Could you check a few things on this drawing? It's one solid part, dimensions in mm from its lowest x, y, z. Give positions to 0.01 mm unless a question says otherwise; leave off trailing zeros. Write each loop counter-clockwise with the first axis right and the second up, starting at its lowest first coordinate (ties: lowest second). Pieces come first, ordered by that corner, then holes. Notation, with made-up numbers: M -32,-17 L -11,-17 A16 cw -11,8 Z; hole C 48,52 d4. An arc over 180 degrees is marked long. Write each question's results on one line, items separated by ' | '.
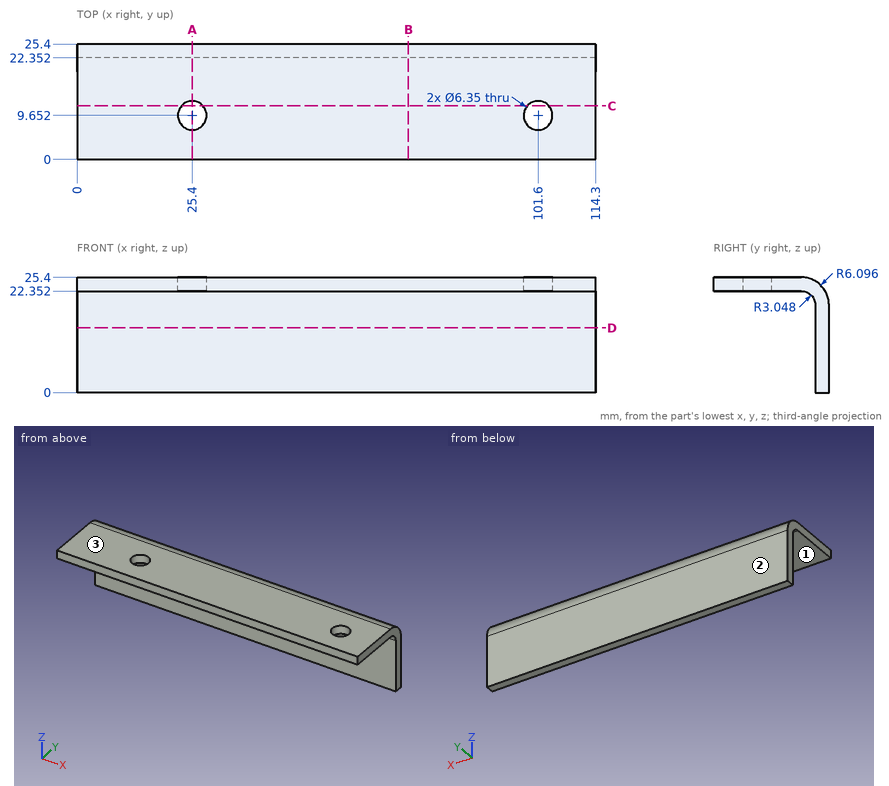
Item 1: I'm going to push flat-ended pins straight in: pin 1 (9.5 mm diameter, centred on x = 84.5, y = 8.5, fed in from -Z); pin 2 (10 mm diameter, centred on x = 42, z = 10, fed in from -Y); pin 3 (12 mm diameter, centred on x = 48.5, y = 16, fed in from -Z); pin 4 (5.5 mm diameter, centred on x = 101.6, y = 9.652, fed in from -Z). Where does each tip first touch, or does it pass through?
Geometry says:
pin 1: stops at z = 22.35 | pin 2: stops at y = 22.35 | pin 3: stops at z = 20.73 | pin 4: passes through
Item 2: I want a section at C-C, the plane y = 11.75. Please give me the cut outline in (x, z), and give its area (3 significant figures).
Geometry says:
outline: M 0,22.35 L 23.02,22.35 L 23.02,25.4 L 0,25.4 Z; M 27.78,22.35 L 99.22,22.35 L 99.22,25.4 L 27.78,25.4 Z; M 103.98,22.35 L 114.3,22.35 L 114.3,25.4 L 103.98,25.4 Z | area: 319 mm2
Item 3: If I drill on line 1 (Y direction, x = 89, z = 7.5); line 2 (Y direction, x = 25.4, z = 23.25); line 3 (Y direction, x = 25.4, z = 24.7), over which ranges is the centre line in solid material (lowest first)? Write a range as from..to.
Geometry says:
line 1: y = 22.35..25.4 | line 2: y = 0..6.48, 12.83..23.95 | line 3: y = 0..6.48, 12.83..22.14
Item 4: I want a section at A-A, the plane x = 25.4. Please give me the cut outline in (y, z).
Geometry says:
outline: M 0,22.35 L 6.48,22.35 L 6.48,25.4 L 0,25.4 Z; M 12.83,22.35 L 19.3,22.35 A3.05 cw 22.35,19.3 L 22.35,0 L 25.4,0 L 25.4,19.3 A6.1 ccw 19.3,25.4 L 12.83,25.4 Z
Item 5: Thinking about a two-plate mould opening in Z: for the marked faces 1, 2 and 3, which applies, +Z half, -Z half, draft (parallel to the pull), parting line (faces both ways), or undercut?
Geometry says:
face 1: -Z half | face 2: draft | face 3: +Z half
Item 6: I want a section at B-B, the plane x = 73. Please give me the cut outline in (y, z), and give its area (3 significant figures).
Geometry says:
outline: M 0,22.35 L 19.3,22.35 A3.05 cw 22.35,19.3 L 22.35,0 L 25.4,0 L 25.4,19.3 A6.1 ccw 19.3,25.4 L 0,25.4 Z | area: 140 mm2
Item 7: I want a section at D-D, the plane z = 14.25. Please give me the cut outline in (x, y).
Geometry says:
outline: M 0,22.35 L 114.3,22.35 L 114.3,25.4 L 0,25.4 Z
